```python
from build123d import *

# Parameters (mm, degrees)
TAGLIO_ESTRUSIONE1_REACH    = 180.821
FORO_20_0_20_1_AT_2_COUNT   = 2
FORO_20_0_20_1_AT_2_PITCH   = 86
RIPETIZIONECIRCOLARE3_COUNT = 4
FORO_20_0_20_3_D            = 20
SCHIZZO12_W                 = 20
SCHIZZO12_H                 = 20
TAGLIO_ESTRUSIONE2_DEPTH    = 189.925496552


with BuildPart() as part:
    # Schizzo1 → Rivoluzione1 (revolve)
    with BuildSketch(Plane.XY, mode=Mode.PRIVATE) as rivoluzione1_sk:
        with BuildLine():
            Line((-108, 44.4), (-57, 44.4))
            ThreePointArc((-57, 44.4), (-58.010409132, 13.995706364), (-31, 0))
            Line((-31, 0), (-31, -48.6))
            Line((-31, -48.6), (-40, -48.6))
            Line((-40, -48.6), (-40, -3.6))
            ThreePointArc((-40, -3.6), (-61.529931917, 9.694522059), (-67, 34.4))
            Line((-67, 34.4), (-108, 34.4))
            Line((-108, 34.4), (-108, 44.4))
        make_face()
    revolve(rivoluzione1_sk.sketch.rotate(Axis((0, 66.063782364, 0), (0, -1, 0)), 270), axis=Axis((0, 66.063782364, 0), (0, -1, 0)))

    # Schizzo2 → Taglio-Estrusione1 (cut, up to next)
    with BuildSketch(Plane(origin=(0, 44.4, 0), x_dir=(1, 0, 0), z_dir=(0, 1, 0)), mode=Mode.PRIVATE) as taglio_estrusione1_sk1:
        with BuildLine():
            Line((-10, 80.5), (-10, 135.944022788))
            ThreePointArc((-10, 135.944022788), (0, 145.944022788), (10, 135.944022788))
            Line((10, 135.944022788), (10, 80.5))
            ThreePointArc((10, 80.5), (0, 70.5), (-10, 80.5))
        make_face()
    taglio_estrusione1_tool1 = extrude(taglio_estrusione1_sk1.sketch, amount=-TAGLIO_ESTRUSIONE1_REACH, mode=Mode.PRIVATE) & part.part
    taglio_estrusione1 = taglio_estrusione1_tool1.solids().sort_by_distance((0, 44.4, -108.222011))[0]
    add(taglio_estrusione1, mode=Mode.SUBTRACT)

    # Schizzo4 → Foro _20.0 _20_-1 (revolve, cut)
    with BuildSketch(Plane(origin=(-60.811183182, 44.4, -60.811183182), x_dir=(0, 0, 1), z_dir=(1, 0, 0))):
        Polygon((0, 0), (0, 41.00860619), (10, 35), (10, 0), align=None)
    foro_20_0_20_1 = revolve(axis=Axis((-60.811183182, 50.75, -60.811183182), (0, -1, 0)), mode=Mode.SUBTRACT)

    # Foro _20.0 _20_-1 at 2: Foro _20.0 _20_-1 ×2
    with Locations(*[Vector(0.7071067811865489, 0, 0.7071067811865462) * (i * FORO_20_0_20_1_AT_2_PITCH) for i in range(1, FORO_20_0_20_1_AT_2_COUNT)]):
        add(foro_20_0_20_1, mode=Mode.SUBTRACT)

    # RipetizioneCircolare3: Taglio-Estrusione1, Foro _20.0 _20_-1 ×4 about axis
    ripetizionecircolare3_axis = Axis((0, 0, 0), (0, 1, 0))
    add([taglio_estrusione1.rotate(ripetizionecircolare3_axis, i * 360 / RIPETIZIONECIRCOLARE3_COUNT) for i in range(1, RIPETIZIONECIRCOLARE3_COUNT)], mode=Mode.SUBTRACT)
    add([foro_20_0_20_1.rotate(ripetizionecircolare3_axis, i * 360 / RIPETIZIONECIRCOLARE3_COUNT) for i in range(1, RIPETIZIONECIRCOLARE3_COUNT)], mode=Mode.SUBTRACT)

    # RipetizioneCircolare3 copy 1 sketch → RipetizioneCircolare3 copy 1 (revolve, cut)
    with BuildSketch(Plane(origin=(0, 44.4, 0), x_dir=(1, 0, 0), z_dir=(0, 0, -1))):
        Polygon((0, 0), (0, 41.00860619), (10, 35), (10, 0), align=None)
    revolve(axis=Axis((0, 50.75, 0), (0, -1, 0)), mode=Mode.SUBTRACT)

    # RipetizioneCircolare3 copy 2 sketch → RipetizioneCircolare3 copy 2 (revolve, cut)
    with BuildSketch(Plane(origin=(0, 44.4, 0), x_dir=(0, 0, -1), z_dir=(-1, 0, 0))):
        Polygon((0, 0), (0, 41.00860619), (10, 35), (10, 0), align=None)
    revolve(axis=Axis((0, 50.75, 0), (0, -1, 0)), mode=Mode.SUBTRACT)

    # RipetizioneCircolare3 copy 3 sketch → RipetizioneCircolare3 copy 3 (revolve, cut)
    with BuildSketch(Plane(origin=(0, 44.4, 0), x_dir=(-1, 0, 0), z_dir=(0, 0, 1))):
        Polygon((0, 0), (0, 41.00860619), (10, 35), (10, 0), align=None)
    revolve(axis=Axis((0, 50.75, 0), (0, -1, 0)), mode=Mode.SUBTRACT)

    # Foro _20.0 _20_-3 (through all)
    with Locations(Plane(origin=(40, 0, 0), x_dir=(0, 0, -1), z_dir=(1, 0, 0))):
        with Locations((0, -28.6)):
            Hole(FORO_20_0_20_3_D / 2)

    # Schizzo12 → Taglio-Estrusione2 (cut, through all)
    with BuildSketch(Plane(origin=(0, 0, -40), x_dir=(-1, 0, 0), z_dir=(0, 0, -1))):
        with Locations((0, -38.6)):
            Rectangle(SCHIZZO12_W, SCHIZZO12_H)
    extrude(amount=-TAGLIO_ESTRUSIONE2_DEPTH, mode=Mode.SUBTRACT)


solid = part.part
```
Input: part model. Units: mm. Frame: model coordinates. A direction names the side the tool comes from. Give positions to 0.01 mm unless a question says otherwise; leave off trailing zeros. Write each loop counter-clockwise with the first axis right and the second up, starting at its lowest first coordinate (ties: lowest second). Pieces come first, ordered by that corner, then holes. Notation, with made-up numbers: (81, 2) - (140, 2) arc R31 cw to (140, 27) - close; hole circle Ø8 at (74.5, 15). An arc over 180 degrees is marked (long way). Write item = value, one per line. Start each with the question number.
1. Section query B-B, the plane z = -74.5. Output: boundary loops of the cut face in (x, y), then the cut area to 3 significant figures.
2. Section query A-A, the plane x = 0. Output: boundary loops of the cut face in (y, z), then the cut area to 3 significant figures.
3. Mould query, pull axis Y, two halves, no side actions, for faces 1 (the flat face through (46, 44.4, 46)), 2 (the flat face through (-10, -39, 34)), 3 (the cylindrical face through (34.607, -32.43, 9.237)). Classes: released by +Y, released by -Y, zero draft, split by the parting line, or undercut.
4. Section query C-C, the plane x = 86.5. Output: boundary loops of the cut face in (y, z), then the cut area to 3 significant figures.
5. Ray query, L1, parallel to X at y = -14, z = 0; L2, parallel to Y at x = -34.25, z = 0; L3, parallel to Y at x = -95, z = 12. Return the intervals inside material, ascending.
6. First-contact query: pin 1 Ø8 at (x, z) = (-48, 36.5) entering from -Y; pin 2 Ø3 at (y, z) = (-41, -32.5) entering from +X; pin 3 Ø3 at (y, z) = (-35, -32.5) entering from -X; pin 4 Ø23 at (x, z) = (60.81, -60.81) entering from +Y. Flat tips, straight axial feed; report the tip coordinate or a pass-through.
7. Access query for faces 4 (the flat face through (10, 39, 94)), 5 (the cylindrical face through (15.32, -25.79, 36.95)), 6 (the flat face through (-94, 39, 10)). Directions: +Z, -Z, +X, -X, +Y, -Y. A direction counts if a zero-diameter tool reaches every point of the face in a straight line with its end or side. Return the directions, or none.
8. Section query D-D, the plane y = 4.5. Output: boundary loops of the cut face in (x, z).
Check sheet entries:
q1.outline = (-78.19, 34.4) - (-8, 34.4) - (-8, 44.4) - (-78.19, 44.4) - close; (8, 34.4) - (78.19, 34.4) - (78.19, 44.4) - (8, 44.4) - close
q1.area = 1,400 mm2
q2.outline = (-28.6, -40) - (-3.6, -40) arc R32.5 ccw to (34.4, -67) - (34.4, -70.5) - (44.4, -70.5) - (44.4, -57) arc R28.5 cw to (0, -31) - (-28.6, -31) - close; (-28.6, 31) - (0, 31) arc R28.5 cw to (44.4, 57) - (44.4, 70.5) - (34.4, 70.5) - (34.4, 67) arc R32.5 ccw to (-3.6, 40) - (-28.6, 40) - close
q2.area = 1,230 mm2
q3.face_1 = released by +Y
q3.face_2 = zero draft
q3.face_3 = undercut
q4.outline = (34.4, -64.67) - (44.4, -64.67) - (44.4, -10) - (34.4, -10) - close; (34.4, 10) - (44.4, 10) - (44.4, 64.67) - (34.4, 64.67) - close
q4.area = 1,090 mm2
q5.L1 = -40 to -31, 31 to 40
q5.L2 = -48.6 to -38.6, -18.6 to -0.09
q5.L3 = 34.4 to 44.4
q6.pin_1 = 3.94
q6.pin_2 = 25.28
q6.pin_3 = -25.28
q6.pin_4 = 44.4
q7.face_4 = +Z, +Y, -Y
q7.face_5 = -Y
q7.face_6 = -X, +Y, -Y
q8.outline = circle Ø113.86 at (0, 0); hole circle Ø97.89 at (0, 0)
